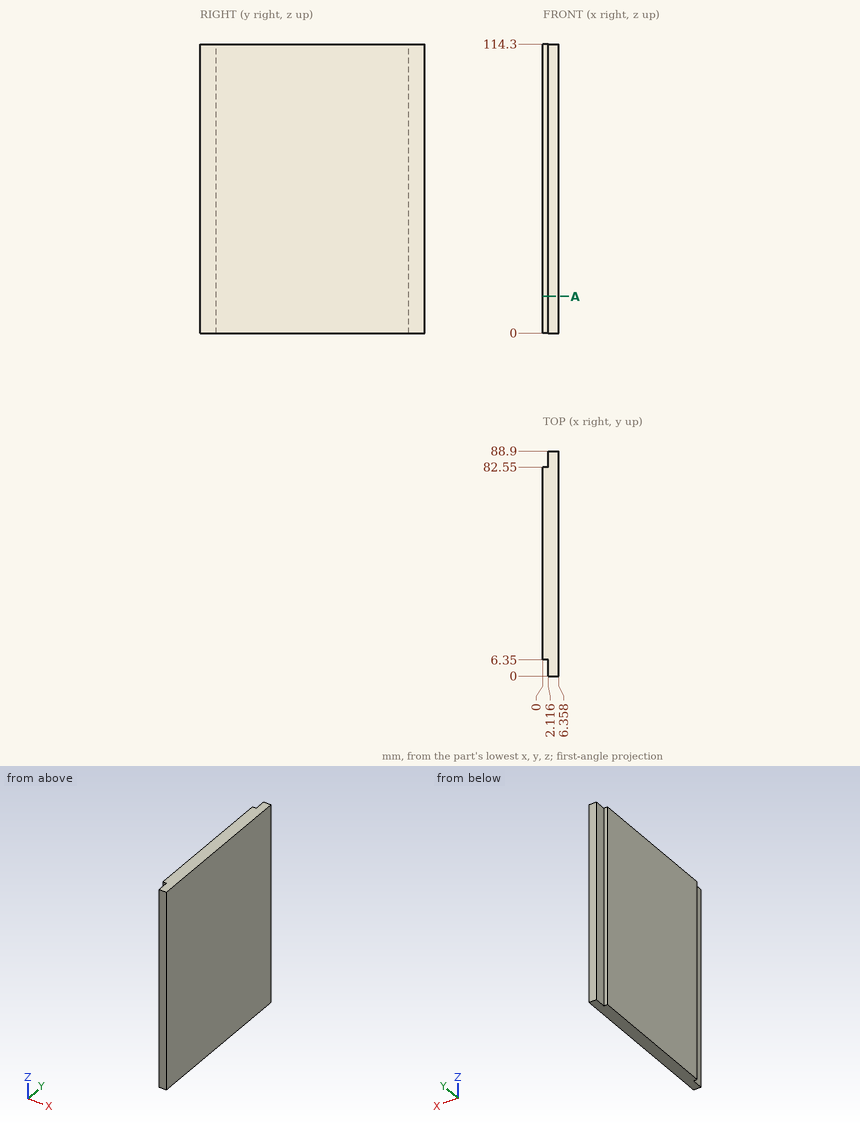
The drawing under review shows one solid part. Ordinate dimensions are in mm from its lowest x, y, z. Give positions to 0.01 mm unless a question says otherwise; leave off trailing zeros. Loops run counter-clockwise (first coordinate to the right, second up) from the corner with the lowest first, then second, coordinate; pieces in that order, holes last. Notation, with made-up numbers: M 12,27 L 26,27 A32 ccw 26,59 Z; hole C 6,73.5 d2. An arc over 180 degrees is marked long. Return JSON: item names as keys, results as strings. Group by question number.
Item 1: For probe 1 along Y at (x, z) = (1.75, 68); probe 2 along X at (y, z) = (4, 48), list the stretches that pass through material, from the lowest coordinate up.
Item 2: Insertion check: pin 1 Ø1.9 at (y, z) = (87, 70) entering from -X; pin 2 Ø2.5 at (x, z) = (0.5, 47) entering from -Y. Each pin has a flat end and moves straight along its axis. Give the tip position at first contact, or say it passes through.
Item 3: We need section A-A (z = 14.5). Give the boundary of the cut face in (x, y), and give its area (3 significant figures).
Output:
{
 "1": {"probe 1": "y = 6.35 to 82.55", "probe 2": "x = 2.12 to 6.36"},
 "2": {"pin 1": "stops at x = 2.12", "pin 2": "stops at y = 6.35"},
 "3": {"outline": "M 0,6.35 L 2.12,6.35 L 2.12,0 L 6.36,0 L 6.36,88.9 L 2.12,88.9 L 2.12,82.55 L 0,82.55 Z", "area": "538 mm^2"}
}
